```python
from build123d import *

# Parameters (mm, degrees)
F1_DEPTH    = 25.4
F3_DEPTH    = 25.4
F4_T1_DEPTH = 159.8348336794
F4_T3_DEPTH = 160.173130017
F4_T6_ANGLE = 219.4963428168


# Not quite as in the source:
# - a fillet or chamfer that OpenCascade refuses, or shapes differently, is made with other operations: its cross-section is extruded or revolved along the edge and cut away or added


with BuildPart() as f1:
    # F0 (on Front) → F1 (new body)
    with BuildSketch(Plane.XZ):
        with BuildLine():
            Line((76.4282107728, 0), (0, 76.1886239052))
            Line((0, 76.1886239052), (-75.9497880936, 0))
            ThreePointArc((-75.9497880936, 0), (0.2392113396, -76.2787980571), (76.4282107728, 0))
        make_face()
    extrude(amount=F1_DEPTH)

    # F2 (on Front) → F3 (cut)
    with BuildSketch(Plane.XZ):
        with BuildLine():
            Line((61.6340054605, 0), (0, 62.5749826431))
            Line((0, 62.5749826431), (-63.5303258896, 0))
            ThreePointArc((-63.5303258896, 0), (-0.9481602145, -62.9010402783), (61.6340054605, 0))
        make_face()
    extrude(amount=F3_DEPTH, mode=Mode.SUBTRACT)

    # F4: chamfer of 10.16 on 3 edges, made by hand

    # F4_s2 → F4_t1 (cut)
    with BuildSketch(Plane(origin=(56.5405950538, 0, 56.7183956672), x_dir=(0, 1, 0), z_dir=(-0.7059958535, 0, -0.7082159662))):
        Polygon((-15.24, -53.7888525608), (-25.4, -43.6288525608), (-25.4, -53.7888525608), align=None)
    extrude(amount=F4_T1_DEPTH, mode=Mode.SUBTRACT)

    # F4_s4 → F4_t3 (cut)
    with BuildSketch(Plane(origin=(56.8385652176, 0, -56.6603878972), x_dir=(0, 1, 0), z_dir=(-0.7082159662, 0, 0.7059958535))):
        Polygon((-15.24, -53.9579998959), (-25.4, -43.7979998959), (-25.4, -53.9579998959), align=None)
    extrude(amount=F4_T3_DEPTH, mode=Mode.SUBTRACT)

    # F4_s5 → F4_t6 (revolve, cut)
    with BuildSketch(Plane(origin=(-0.0012303148, 0, -0.0034270544), x_dir=(0, 1, 0), z_dir=(0.3378866803, 0, 0.9411867994))):
        Polygon((-15.24, 75.9335858363), (-25.4, 65.7735858363), (-25.4, 75.9335858363), align=None)
    revolve(axis=Axis((0.2392113396, -25.4, -0.0897457666), (0, -1, 0)), revolution_arc=F4_T6_ANGLE, mode=Mode.SUBTRACT)


solid = f1.part
```
Check sheet for the modelled part. Datum: model origin and axes. Units: mm. A direction names the side the tool comes from. Coordinates: 2 decimals unless noted, no trailing zeros. Write each loop counter-clockwise with the first axis right and the second up, starting at its lowest first coordinate (ties: lowest second). Pieces come first, ordered by that corner, then holes. Notation, with made-up numbers: M 72.25,62.5 L 98.25,62.5 A22 cw 98.25,78.5 Z; hole C -40,-36.5 d10. An arc over 180 degrees is marked long. Write item = value, one per line. Start each with the question number.
1. Thickness scan on probe 1 along Z at (x, y) = (-27, -15); probe 2 along X at (y, z) = (-9, 29); probe 3 along X at (y, z) = (-4.5, -43.5). Record the ranges inside material, lowest first.
2. Tool access check on faces 1 (the cylindrical face through (-2.329, -12.522, -62.886)), 2 (the flat face through (-33.896, -20.249, 35.091)). Record the directions out of +Z, -Z, +X, -X, +Y, -Y that give a thin tool (end or side, any length) a straight path to the whole face; none if there is none.
3. Sectioned sample at A-A (z = 16.5). Record the cut outline in (x, y), then the cut area to 3 significant figures.
4. Mould release check, pull along Z, two halves, no side actions. Record for faces 3 (the flat face through (31.25, -12.52, 30.85)), 4 (the flat face through (11, 0, -62)), 5 (the flat face through (38.75, -7.51, 37.56)): pulls with the +Z half, pulls with the -Z half, needs draft (parallel to the pull), parting line crosses it, or undercut.
5. Sectioned sample at C-C (z = 35). Record the cut outline in (x, y), then the cut area to 3 significant figures.
6. Go/stop test with flat-tipped pins: pin 1 (1 mm diameter, centred on x = -51, y = -23, fed in from +Z); pin 2 (10 mm diameter, centred on y = -18, z = 33.5, fed in from -X); pin 3 (4 mm diameter, centred on y = -11.5, z = 32.5, fed in from +X). Record where each tip stops, or that it passes through.
The answers:
q1.probe_1 = -71.24 to -57.22, 35.98 to 49.1
q1.probe_2 = -47.04 to -34.09, 33.07 to 47.34
q1.probe_3 = -62.37 to -46.25, 44.35 to 62.85
q2.face_1 = +Y, -Y
q2.face_2 = +Z, -X, -Y
q3.outline = M -59.5,-15.24 L -46.78,-24.25 L -46.78,0 L -59.5,0 Z; M 45.38,-25.4 L 45.49,-25.4 L 59.88,-15.24 L 59.88,0 L 45.38,0 Z
q3.area = 546 mm²
q4.face_3 = undercut
q4.face_4 = needs draft
q4.face_5 = pulls with the +Z half
q5.outline = M -41.06,-15.24 L -28,-24.49 L -28,0 L -41.06,0 Z; M 27.16,-25.24 L 41.32,-15.24 L 41.32,0 L 27.16,0 Z
q5.area = 546 mm²
q6.pin_1 = 14.9
q6.pin_2 = -46.71
q6.pin_3 = 45.83
